Could you check a few things on this drawing? It's one solid part, dimensions in mm from its lowest x, y, z. Round coordinates to 2 decimals unless told otherwise and drop trailing zeros. Loops run counter-clockwise (first coordinate to the right, second up) from the corner with the lowest first, then second, coordinate; pieces in that order, holes last. Notation, with made-up numbers: M -24.75,31 L 17.25,31 A10 cw 17.25,47 Z; hole C 20.5,78 d4. An arc over 180 degrees is marked long. Return JSON: item names as keys, results as strings.
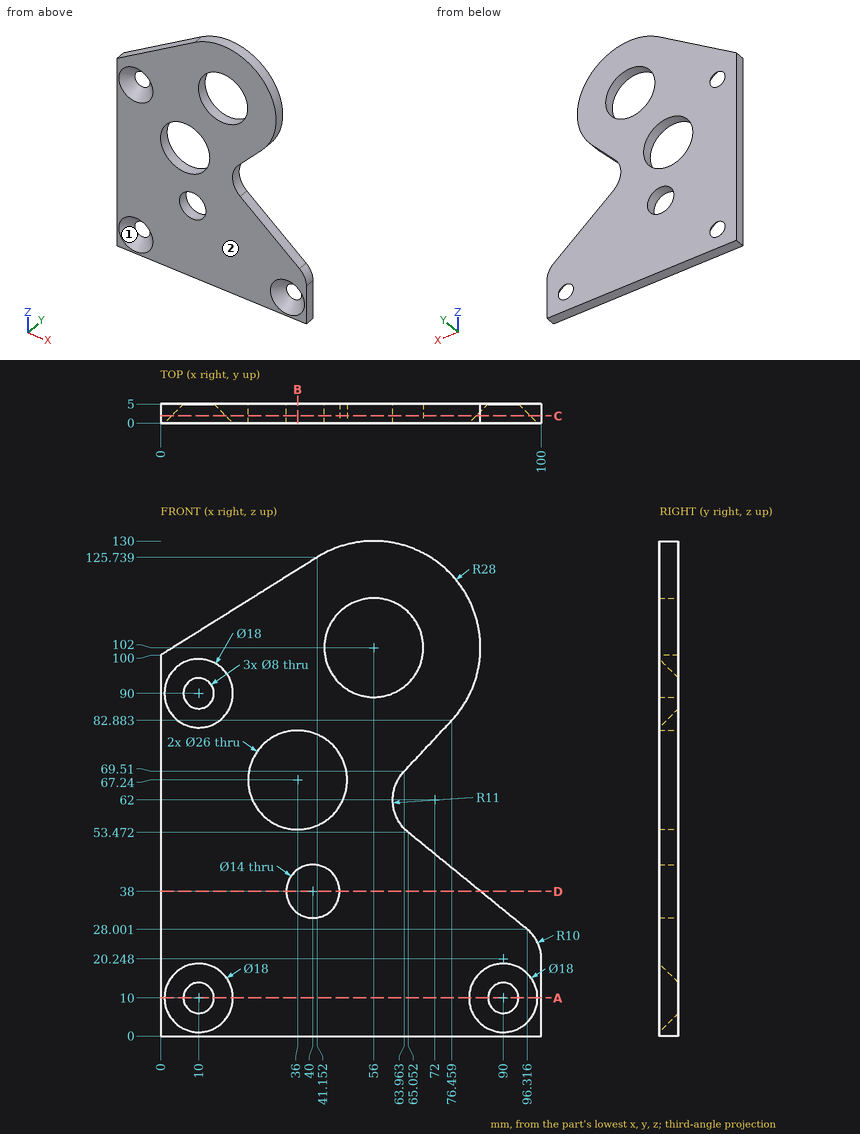
Q1. Suppose I cut it at C-C, the plane y = 1.9. Please give me the cut outline in (x, z), plus the area to 3 significant figures.
Results:
{"outline": "M 0,0 L 100,0 L 100,20.25 A10 ccw 96.32,28 L 65.05,53.47 A11 cw 63.96,69.51 L 76.46,82.88 A28 ccw 41.15,125.74 L 0,100 Z; hole C 10,10 d14.2; hole C 10,90 d14.2; hole C 36,67.24 d26; hole C 40,38 d14; hole C 56,102 d26; hole C 90,10 d14.2", "area": "8,110 mm2"}
Q2. If I drill on line 1 along Z through (x, y) = (56, 2.1); line 2 along Z through (x, y) = (40, 1); line 3 along Z through (x, y) = (65.5, 4.1) (1 decimal), over which ranges is the centre line in solid material (lowest first)?
Results:
{"line 1": "z = 0 to 89, 115 to 130", "line 2": "z = 0 to 31, 45 to 54.87, 79.61 to 125.02", "line 3": "z = 0 to 53.1, 71.2 to 93.1, 110.9 to 128.3"}
Q3. Suppose I cut it at D-D, the plane z = 38. Please give me the cut outline in (x, y), plus the area to 3 significant figures.
Results:
{"outline": "M 0,0 L 33,0 L 33,5 L 0,5 Z; M 47,0 L 84.04,0 L 84.04,5 L 47,5 Z", "area": "350 mm2"}
Q4. I'm going to push flat-ended pins straight in: pin 1 Ø2 at (y, z) = (2.5, 47.5) entering from +X; pin 2 Ø1.5 at (x, y) = (14, 2.5) entering from +Z (1 decimal); pin 3 Ø6.5 at (x, z) = (10, 10) entering from +Y; pin 4 Ø2 at (y, z) = (2.5, 25.5) entering from +X. Where does each tip first touch, or does it pass through?
Results:
{"pin 1": "stops at x = 73.61", "pin 2": "stops at z = 109.2", "pin 3": "passes through", "pin 4": "stops at x = 99.05"}
Q5. Suppose I cut it at A-A, the plane z = 10. State how many separate pieces and enclosed holes the cut face has, plus the area to 3 significant figures.
Results:
{"separate pieces": "3", "enclosed holes": "0", "area": "370 mm2"}
Q6. Suppose I cut it at B-B, the plane x = 36. Please give me the cut outline in (y, z) (1 decimal).
Results:
{"outline": "M 0,0 L 5,0 L 5,32.3 L 0,32.3 Z; M 0,43.7 L 5,43.7 L 5,54.2 L 0,54.2 Z; M 0,80.2 L 5,80.2 L 5,122.5 L 0,122.5 Z"}
Q7. Thinking about a two-plate mould opening in Z: for the marked faces 1 and 2, which applies, pulls with the +Z half, pulls with the -Z half, needs draft (parallel to the pull), parting line crosses it, or undercut?
Results:
{"face 1": "undercut", "face 2": "needs draft"}
